from build123d import *


with BuildPart() as part:
    # Sweep1: sweep along a path in Sketch4
    with BuildLine(Plane.XY) as sweep1_path:
        Line((0, 0), (0, 40.3))
        ThreePointArc((0, 40.3), (1.815937957, 44.684062043), (6.2, 46.5))
        Line((6.2, 46.5), (15.5, 46.5))
    # Sketch3 → Sweep1 (sweep)
    with BuildSketch(Plane(origin=(0, 0, 0), x_dir=(1, 0, 0), z_dir=(0, 1, 0))):
        Polygon((0, 0.866025404), (-0.75, 0.433012702), (-0.75, -0.433012702), (0, -0.866025404), (0.75, -0.433012702), (0.75, 0.433012702), align=None)
    sweep(path=sweep1_path.line)


solid = part.part
Source: CAD feature listing. Evaluate the final solid. Frame: model axes, mm. A direction names the side the tool comes from. Round coordinates to 2 decimals unless told otherwise and drop trailing zeros. Loops run counter-clockwise (first coordinate to the right, second up) from the corner with the lowest first, then second, coordinate; pieces in that order, holes last.
Q1. First-contact query: P1, Ø0.7, axis at y = 19, z = 0, coming from the +X side; P2, Ø3, axis at x = 2, y = 20.5, coming from the +Z side. Flat tips, straight axial feed; report the tip coordinate or a pass-through.
Q2. Ray query, line 1 (Y direction, x = 7, z = -0.1); line 2 (X direction, y = 35.5, z = 0.1). Return the intervals inside material, ascending.
Q3. Section C-C, the plane y = 4.5. Return loops of the section in (x, z), plus the area to 3 significant figures.
Q4. Access query for faces 1 (the face through (0.75, 20, 0)), 2 (the face through (-0.75, 20, 0)). Directions: +Z, -Z, +X, -X, +Y, -Y. A direction counts if a zero-diameter tool reaches every point of the face in a straight line with its end or side. Return the directions, or none.
Q5. Section B-B, the plane x = 8. Return loops of the section in (y, z).
Q6. Section A-A, the plane z = 0. Return loops of the section in (x, y).
Solutions:
1. P1: stops at x = 0.75
1. P2: stops at z = 0.58
2. line 1: y = 45.75 to 47.25
2. line 2: x = -0.75 to 0.75
3. outline: (-0.75, -0.43) - (0, -0.87) - (0.75, -0.43) - (0.75, 0.43) - (0, 0.87) - (-0.75, 0.43) - close
3. area: 1.95 mm2
4. face 1: +Z, -Z, +X, -Y
4. face 2: +Z, -Z, -X, +Y, -Y
5. outline: (45.75, -0.43) - (46.5, -0.87) - (47.25, -0.43) - (47.25, 0.43) - (46.5, 0.87) - (45.75, 0.43) - close
6. outline: (-0.75, 0) - (0.75, 0) - (0.75, 40.3) arc R5.45 cw to (6.2, 45.75) - (15.5, 45.75) - (15.5, 47.25) - (6.2, 47.25) arc R6.95 ccw to (-0.75, 40.3) - close
